Input: part model. Units: mm. Frame: model coordinates. A direction names the side the tool comes from. Coordinates: 2 decimals unless noted, no trailing zeros. Order: outer loops, then holes, each group sorted by start corner. A loop starts at its lowest first (then second) coordinate and runs counter-clockwise, first axis right, second up. Notation, with made-up numbers: (74.25, 20.5) - (103.25, 20.5) arc R16 cw to (103.25, 28.5) - close; hole circle Ø6 at (85.25, 1.5). An arc over 180 degrees is marked (long way). Use a Markdown table: item, result. Add a question column.
from build123d import *

# Parameters (mm, degrees)
F0_W     = 33
F0_H     = 29
F1_DEPTH = 2
F2_W     = 33
F2_H     = 29
F2_W_2   = 31
F2_H_2   = 27
F3_DEPTH = 2
F4_W     = 25
F4_H     = 21
F4_W_2   = 23
F4_H_2   = 19
F5_DEPTH = 2
F6_R     = 4.5
F6_R_2   = 3.5
F7_DEPTH = 2


with BuildPart() as f1:
    # F0 (on Top) → F1 (new body)
    with BuildSketch(Plane.XY):
        Rectangle(F0_W, F0_H)
    extrude(amount=F1_DEPTH)

    # F2 (on face) → F3 (join)
    with BuildSketch(Plane.XY.offset(2)):
        Rectangle(F2_W, F2_H)
        Rectangle(F2_W_2, F2_H_2, mode=Mode.SUBTRACT)
    extrude(amount=F3_DEPTH)

    # F4 (on face) → F5 (join)
    with BuildSketch(Plane.XY.offset(2)):
        Rectangle(F4_W, F4_H)
        Rectangle(F4_W_2, F4_H_2, mode=Mode.SUBTRACT)
    extrude(amount=F5_DEPTH)

    # F6 (on face) → F7 (join)
    with BuildSketch(Plane.XY.offset(2)):
        with Locations((-3, -6)):
            Circle(F6_R)
        with Locations((-3, -6)):
            Circle(F6_R_2, mode=Mode.SUBTRACT)
    extrude(amount=F7_DEPTH)


solid = f1.part
1) Cut plane D-D (y = -0.5). Return the cut outline in (x, z).
2) Pull-direction query (X, two-part tool) for faces 1 (the flat face through (0, 0, 2)), 2 (the flat face through (16.5, 0, 2)), 3 (the flat face through (0, 14.5, 2)); classes: pulls with the +X half, pulls with the -X half, needs draft (parallel to the pull), parting line crosses it, or undercut.
3) Cut plane C-C (x = 2.5). Return the cut outline in (y, z).
4) Reachability of faces 4 (the flat face through (-16.5, 0, 2)), 5 (the flat face through (0, -13.5, 3)) from +Z, -Z, +X, -X, +Y, -Y: full face, straight path, thin tool, end or side. Return the list, or none.
5) Contact query for flat-ended pins moving along their axis: P1, Ø13.5, axis at x = 5, y = -5, coming from the +Z side; P2, Ø3.5, axis at x = -3, y = -5, coming from the +Z side. Output: stop coordinate, or through.
6) Cut plane B-B (y = -6). Return the cut outline in (x, z).
7) Cut plane A-A (z = 3.1). Return the cut outline in (x, y), and give its area (3 significant figures).
8) Material intervals for L1, parallel to X at y = -6, z = 3; L2, parallel to Y at x = -3, z = 2.75; L3, parallel to Y at x = 8, z = 2.9, sorted ascending.
Computed:
| question | item | result |
|---|---|---|
| 1 | outline | (-16.5, 0) - (16.5, 0) - (16.5, 4) - (15.5, 4) - (15.5, 2) - (12.5, 2) - (12.5, 4) - (11.5, 4) - (11.5, 2) - (-11.5, 2) - (-11.5, 4) - (-12.5, 4) - (-12.5, 2) - (-15.5, 2) - (-15.5, 4) - (-16.5, 4) - close |
| 2 | face 1 | undercut |
| 2 | face 2 | pulls with the +X half |
| 2 | face 3 | needs draft |
| 3 | outline | (-14.5, 0) - (14.5, 0) - (14.5, 4) - (13.5, 4) - (13.5, 2) - (10.5, 2) - (10.5, 4) - (9.5, 4) - (9.5, 2) - (-9.5, 2) - (-9.5, 4) - (-10.5, 4) - (-10.5, 2) - (-13.5, 2) - (-13.5, 4) - (-14.5, 4) - close |
| 4 | face 4 | +Z, -Z, -X, +Y, -Y |
| 4 | face 5 | +Z |
| 5 | P1 | stops at z = 4 |
| 5 | P2 | stops at z = 2 |
| 6 | outline | (-16.5, 0) - (16.5, 0) - (16.5, 4) - (15.5, 4) - (15.5, 2) - (12.5, 2) - (12.5, 4) - (11.5, 4) - (11.5, 2) - (1.5, 2) - (1.5, 4) - (0.5, 4) - (0.5, 2) - (-6.5, 2) - (-6.5, 4) - (-7.5, 4) - (-7.5, 2) - (-11.5, 2) - (-11.5, 4) - (-12.5, 4) - (-12.5, 2) - (-15.5, 2) - (-15.5, 4) - (-16.5, 4) - close |
| 7 | outline | (-16.5, -14.5) - (16.5, -14.5) - (16.5, 14.5) - (-16.5, 14.5) - close; (-12.5, -10.5) - (12.5, -10.5) - (12.5, 10.5) - (-12.5, 10.5) - close; hole (-15.5, -13.5) - (15.5, -13.5) - (15.5, 13.5) - (-15.5, 13.5) - close; hole (-11.5, -9.5) - (-5.83, -9.5) arc R4.5 cw (long way) to (-0.17, -9.5) - (11.5, -9.5) - (11.5, 9.5) - (-11.5, 9.5) - close; hole circle Ø7 at (-3, -6) |
| 7 | area | 229 mm2 |
| 8 | L1 | x = -16.5 to -15.5, -12.5 to -11.5, -7.5 to -6.5, 0.5 to 1.5, 11.5 to 12.5, 15.5 to 16.5 |
| 8 | L2 | y = -14.5 to -13.5, -10.5 to -9.5, -2.5 to -1.5, 9.5 to 10.5, 13.5 to 14.5 |
| 8 | L3 | y = -14.5 to -13.5, -10.5 to -9.5, 9.5 to 10.5, 13.5 to 14.5 |
